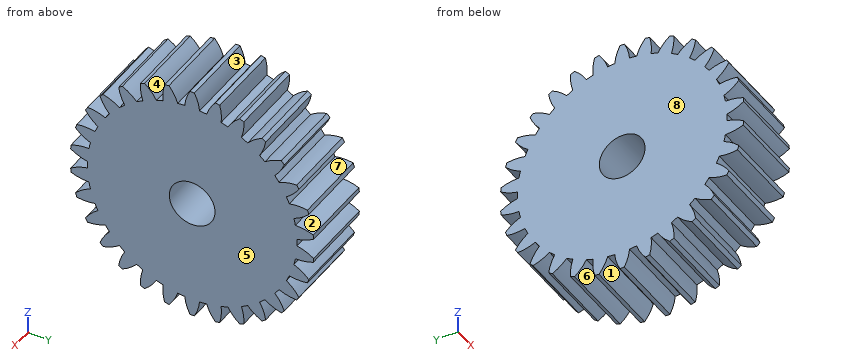
```python
from build123d import *

# Parameters (mm, degrees)
BASPROSKE_W        = 10
BASPROSKE_H        = 16
TOOTHCUT_DEPTH     = 25.738633754
TEETHCUTS_COUNT    = 30
TEETHCUTS_ANGLE    = 348
HUBNEAONESKE_R     = 12.5
HUBNEARONE_DEPTH   = 8.0000508
BORSKE_R           = 3
BORE_DEPTH         = 18.0000508
SKETCH1_R          = 12.5
CUT_EXTRUDE1_DEPTH = 8.0000508


with BuildPart() as part:
    # BasProSke → Base-Revolve (revolve)
    with BuildSketch(Plane(origin=(0, 0, 0), x_dir=(1, 0, 0), z_dir=(0, 1, 0)), mode=Mode.PRIVATE) as base_revolve_sk:
        with Locations((5, 8)):
            Rectangle(BASPROSKE_W, BASPROSKE_H)
    revolve(base_revolve_sk.sketch.rotate(Axis((-10, 0, 0), (1, 0, 0)), 180), axis=Axis((-10, 0, 0), (1, 0, 0)))

    # TooCutSke → ToothCut (cut, through all)
    with BuildSketch(Plane(origin=(0, 0, 0), x_dir=(0, 0, -1), z_dir=(1, 0, 0))):
        with BuildLine():
            ThreePointArc((0.466400716, 13.741086979), (0, 13.749), (-0.466400716, 13.741086979))
            ThreePointArc((-0.466400716, 13.741086979), (-0.819142092, 14.899954875), (-1.3974676, 15.964351834))
            ThreePointArc((-1.3974676, 15.964351834), (0, 16.0254), (1.3974676, 15.964351834))
            ThreePointArc((1.3974676, 15.964351834), (0.819142092, 14.899954875), (0.466400716, 13.741086979))
        make_face()
    toothcut = extrude(amount=TOOTHCUT_DEPTH, mode=Mode.SUBTRACT)

    # TeethCuts: ToothCut ×30 about axis
    teethcuts_axis = Axis((-10, 0, 0), (1, 0, 0))
    for i in range(1, TEETHCUTS_COUNT):
        add(toothcut.rotate(teethcuts_axis, i * TEETHCUTS_ANGLE / (TEETHCUTS_COUNT - 1)), mode=Mode.SUBTRACT)

    # HubNeaOneSke → HubNearOne (add)
    with BuildSketch(Plane.ZY):
        with Locations(Location((0, 0, 0), (0, 0, 180))):
            Circle(HUBNEAONESKE_R)
    extrude(amount=HUBNEARONE_DEPTH)

    # BorSke → Bore (cut, symmetric)
    with BuildSketch(Plane(origin=(0, 0, 0), x_dir=(0, 0, -1), z_dir=(1, 0, 0))):
        with Locations(Location((0, 0, 0), (0, 0, 180))):
            Circle(BORSKE_R)
    extrude(amount=BORE_DEPTH, both=True, mode=Mode.SUBTRACT)

    # Sketch1 → Cut-Extrude1 (cut)
    with BuildSketch(Plane.ZY.offset(8.0000508)):
        Circle(SKETCH1_R)
    extrude(amount=-CUT_EXTRUDE1_DEPTH, mode=Mode.SUBTRACT)


solid = part.part
```
The model under review builds one solid part; all positions refer to its coordinate system, in mm. Face numbers are marked on the shaded views. A direction names the side the tool comes from. Give positions to 0.01 mm unless a question says otherwise; leave off trailing zeros. Write each loop counter-clockwise with the first axis right and the second up, starting at its lowest first coordinate (ties: lowest second). Pieces come first, ordered by that corner, then holes. Notation, with made-up numbers: M 8,-9.75 L 47,-9.75 A29 ccw 47,12.25 Z; hole C 70,-18 d2. An arc over 180 degrees is marked long. Answer in a Markdown table with one row per item.
Item 1: For line 1 along Y through (x, z) = (3, 0); line 2 along Y through (x, z) = (7.5, 15); line 3 along Y through (x, z) = (1, -12), list the stretches that pass through material, from the lowest coordinate up.
Check sheet entries:
| item | result |
|---|---|
| line 1 | -13.75 to -3, 3 to 13.75 |
| line 2 | -3.75 to -2.53, -0.71 to 0.71, 2.53 to 3.75 |
| line 3 | -9.48 to -7.59, -6.71 to 6.71, 7.59 to 9.48 |
Item 2: Add section A-A on z = 0. Give the boundary of the cut face in (x, y), plus the area to 3 significant figures.
Check sheet entries:
| item | result |
|---|---|
| outline | M 0,-13.75 L 10,-13.75 L 10,-3 L 0,-3 Z; M 0,3 L 10,3 L 10,13.75 L 0,13.75 Z |
| area | 215 mm2 |
Item 3: Draft analysis for pull direction Z (two halves, no side actions). For the marked faces 1, 2 and 3, state which applies: +Z half, -Z half, draft (parallel to the pull), parting line (faces both ways), or undercut.
Check sheet entries:
| item | result |
|---|---|
| face 1 | -Z half |
| face 2 | undercut |
| face 3 | +Z half |
Item 4: Tool access review of the marked faces 4, 5, 6, 7 and 8: name each direction out of +Z, -Z, +X, -X, +Y, -Y from which nothing blocks a thin tool from reaching the whole face with its end or side.
Check sheet entries:
| item | result |
|---|---|
| face 4 | +Z, +X, -X |
| face 5 | +Z, -Z, +X, +Y, -Y |
| face 6 | -Z, +X, -X |
| face 7 | +X, -X |
| face 8 | +Z, -Z, -X, +Y, -Y |
Item 5: Add section B-B on z = 9. Give the boundary of the cut face in (x, y).
Check sheet entries:
| item | result |
|---|---|
| outline | M 0,-11.29 L 10,-11.29 L 10,11.29 L 0,11.29 Z |
Item 6: For P1, Ø3, axis at x = 3.5, y = -5, coming from the -Z side; P2, Ø6, axis at x = 1, y = 7.5, coming from the -Z side; P3, Ø3, axis at x = 8, z = 2, coming from the -Y side, all flat-tipped, find the tip position at first contact; note any pin that passes through.
Check sheet entries:
| item | result |
|---|---|
| P1 | z = -15.61 |
| P2 | z = -14.73 |
| P3 | y = -15.94 |
